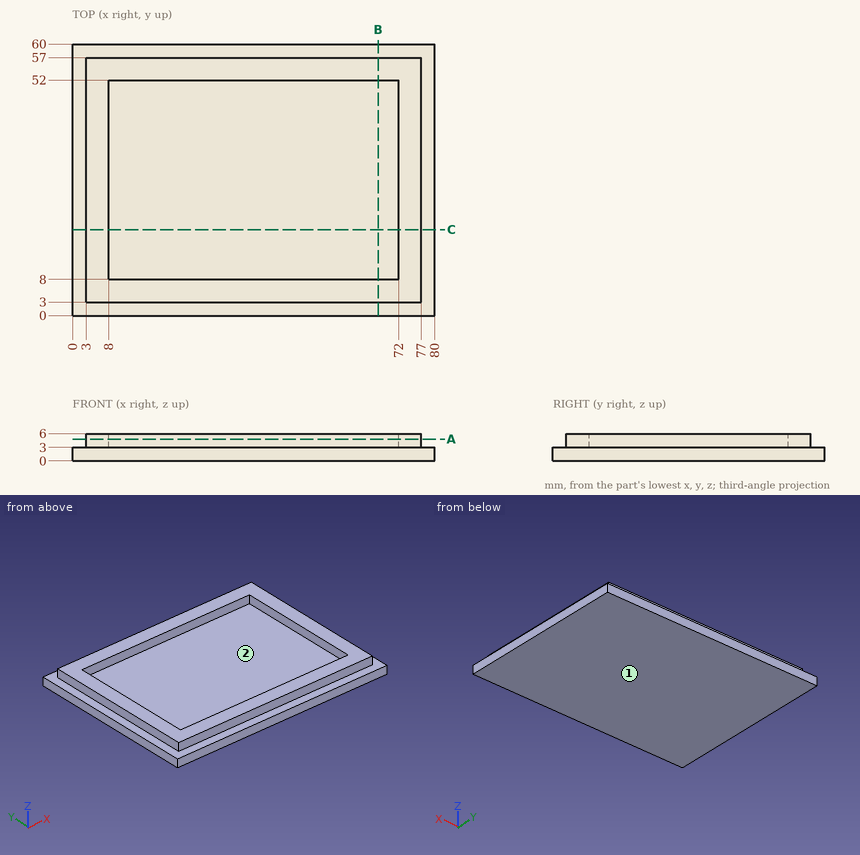
Here's the drawing with two shaded views (mm, measured from the low corner). I have some questions. Give positions to 0.01 mm unless a question says otherwise; leave off trailing zeros. Loops run counter-clockwise (first coordinate to the right, second up) from the corner with the lowest first, then second, coordinate; pieces in that order, holes last. Notation, with made-up numbers: M 88,46.25 L 145,46.25 A24 ccw 145,79.25 Z; hole C 1,-30 d7. An arc over 180 degrees is marked long. Use one line per item in the form item = value. Start each with the question number.
(1) I want a section at C-C, the plane y = 19. Write out the boundary of the cut face in (x, z), and give its area (3 significant figures).
(2) I want a section at A-A, the plane z = 4.8. Write out the boundary of the cut face in (x, y), and give its area (3 significant figures).
(3) Please list where these lines run through material, in increasing order: line 1 (X direction, y = 24, z = 4.35); line 2 (Y direction, x = 10, z = 3.5); line 3 (Z direction, x = 20, y = 28.5).
(4) I'm going to push flat-ended pins straight in: P1, Ø1.5, axis at x = 54, z = 4.5, coming from the -Y side; P2, Ø2.5, axis at y = 18.5, z = 5, coming from the +X side; P3, Ø0.9, axis at y = 20.5, z = 4.5, coming from the -X side. Where does each tip first touch, or does it pass through?
(5) I want a section at B-B, the plane x = 67.5. Write out the boundary of the cut face in (y, z).
(6) Thinking about a two-plate mould opening in X: for the marked faces 1 and 2, which applies, released by +X, released by -X, zero draft, split by the parting line, or undercut?
Worked out:
q1.outline = M 0,0 L 80,0 L 80,3 L 77,3 L 77,6 L 72,6 L 72,3 L 8,3 L 8,6 L 3,6 L 3,3 L 0,3 Z
q1.area = 270 mm²
q2.outline = M 3,3 L 77,3 L 77,57 L 3,57 Z; hole M 8,8 L 72,8 L 72,52 L 8,52 Z
q2.area = 1,180 mm²
q3.line_1 = 3 to 8, 72 to 77
q3.line_2 = 3 to 8, 52 to 57
q3.line_3 = 0 to 3
q4.P1 = 3
q4.P2 = 77
q4.P3 = 3
q5.outline = M 0,0 L 60,0 L 60,3 L 57,3 L 57,6 L 52,6 L 52,3 L 8,3 L 8,6 L 3,6 L 3,3 L 0,3 Z
q6.face_1 = zero draft
q6.face_2 = undercut
